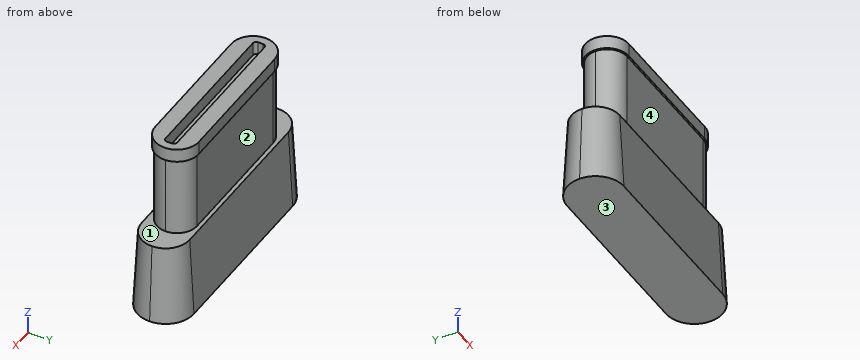
```python
from build123d import *

# Parameters (mm, degrees)
F1_DEPTH  = 2
F3_DEPTH  = 12
F5_DEPTH  = 12
F5_TAPER  = -3
F6_W      = 24
F6_H      = 1.75
F7_DEPTH  = 2
F8_R      = 0.5
F10_DEPTH = 2


with BuildPart() as f1:
    # F0 (on Top) → F1 (new body)
    with BuildSketch(Plane.XY):
        with BuildLine():
            ThreePointArc((0, 2.5), (0.732233047, 0.732233047), (2.5, 0))
            Line((2.5, 0), (22.5, 0))
            ThreePointArc((22.5, 0), (24.267766953, 0.732233047), (25, 2.5))
            ThreePointArc((25, 2.5), (24.267766953, 4.267766953), (22.5, 5))
            Line((22.5, 5), (2.5, 5))
            ThreePointArc((2.5, 5), (0.732233047, 4.267766953), (0, 2.5))
        make_face()
    extrude(amount=-F1_DEPTH)

    # F2 (on face) → F3 (join)
    with BuildSketch(Plane(origin=(0, 0, -2), x_dir=(1, 0, 0), z_dir=(0, 0, -1))):
        with BuildLine():
            ThreePointArc((2.5, 0.5), (0.3786796564, -0.3786796564), (-0.5, -2.5))
            ThreePointArc((-0.5, -2.5), (0.3786796564, -4.6213203436), (2.5, -5.5))
            Line((2.5, -5.5), (22.5, -5.5))
            ThreePointArc((22.5, -5.5), (24.6213203436, -4.6213203436), (25.5, -2.5))
            ThreePointArc((25.5, -2.5), (24.6213203436, -0.3786796564), (22.5, 0.5))
            Line((22.5, 0.5), (2.5, 0.5))
        make_face()
        with BuildLine():
            Line((2.5, 0), (22.5, 0))
            ThreePointArc((22.5, 0), (25, -2.5), (22.5, -5))
            Line((22.5, -5), (2.5, -5))
            ThreePointArc((2.5, -5), (0, -2.5), (2.5, 0))
        make_face(mode=Mode.SUBTRACT)
        with BuildLine():
            ThreePointArc((22.5, -5), (25, -2.5), (22.5, 0))
            Line((22.5, 0), (2.5, 0))
            ThreePointArc((2.5, 0), (0, -2.5), (2.5, -5))
            Line((2.5, -5), (22.5, -5))
        make_face()
    extrude(amount=F3_DEPTH)

    # F4 (on face) → F5 (join)
    with BuildSketch(Plane(origin=(0, 0, -14), x_dir=(1, 0, 0), z_dir=(0, 0, -1))):
        with BuildLine():
            Line((25.5, 1.099999994), (-0.5, 1.099999994))
            ThreePointArc((-0.5, 1.099999994), (-3.0455844081, 0.0455844081), (-4.099999994, -2.5))
            ThreePointArc((-4.099999994, -2.5), (-3.0455844081, -5.0455844081), (-0.5, -6.099999994))
            Line((-0.5, -6.099999994), (25.5, -6.099999994))
            ThreePointArc((25.5, -6.099999994), (28.0455844081, -5.0455844081), (29.099999994, -2.5))
            ThreePointArc((29.099999994, -2.5), (28.0455844081, 0.0455844081), (25.5, 1.099999994))
        make_face()
        with BuildLine():
            ThreePointArc((-3.5, -2.5), (-2.6213203436, -0.3786796564), (-0.5, 0.5))
            Line((-0.5, 0.5), (2.5, 0.5))
            Line((2.5, 0.5), (22.5, 0.5))
            Line((22.5, 0.5), (25.5, 0.5))
            ThreePointArc((25.5, 0.5), (27.6213203436, -0.3786796564), (28.5, -2.5))
            ThreePointArc((28.5, -2.5), (27.6213203436, -4.6213203436), (25.5, -5.5))
            Line((25.5, -5.5), (22.5, -5.5))
            Line((22.5, -5.5), (2.5, -5.5))
            Line((2.5, -5.5), (-0.5, -5.5))
            ThreePointArc((-0.5, -5.5), (-2.6213203436, -4.6213203436), (-3.5, -2.5))
        make_face(mode=Mode.SUBTRACT)
        with BuildLine():
            Line((22.5, 0.5), (2.5, 0.5))
            ThreePointArc((2.5, 0.5), (-0.5, -2.5), (2.5, -5.5))
            Line((2.5, -5.5), (22.5, -5.5))
            ThreePointArc((22.5, -5.5), (25.5, -2.5), (22.5, 0.5))
        make_face()
        with BuildLine():
            Line((2.5, 0.5), (-0.5, 0.5))
            ThreePointArc((-0.5, 0.5), (-2.6213203436, -0.3786796564), (-3.5, -2.5))
            ThreePointArc((-3.5, -2.5), (-2.6213203436, -4.6213203436), (-0.5, -5.5))
            Line((-0.5, -5.5), (2.5, -5.5))
            ThreePointArc((2.5, -5.5), (-0.5, -2.5), (2.5, 0.5))
        make_face()
        with BuildLine():
            Line((25.5, 0.5), (22.5, 0.5))
            ThreePointArc((22.5, 0.5), (25.5, -2.5), (22.5, -5.5))
            Line((22.5, -5.5), (25.5, -5.5))
            ThreePointArc((25.5, -5.5), (27.6213203436, -4.6213203436), (28.5, -2.5))
            ThreePointArc((28.5, -2.5), (27.6213203436, -0.3786796564), (25.5, 0.5))
        make_face()
    extrude(amount=F5_DEPTH, taper=F5_TAPER)

    # F6 (on face) → F7 (cut)
    with BuildSketch(Plane.XY):
        with Locations((12.5, 2.5)):
            Rectangle(F6_W, F6_H)
    extrude(amount=-F7_DEPTH, mode=Mode.SUBTRACT)

    # F8
    f8_edges = [f1.edges().sort_by_distance(p)[0] for p in [
        (0.5, 3.375, -1),
        (0.5, 1.625, -1),
        (24.5, 1.625, -1),
        (24.5, 3.375, -1),
    ]]
    fillet(f8_edges, radius=F8_R)

    # F9 (on face) → F10 (join)
    with BuildSketch(Plane.XY):
        with BuildLine():
            Line((22.5, 5.75), (2.5, 5.75))
            ThreePointArc((2.5, 5.75), (-0.75, 2.5), (2.5, -0.75))
            Line((2.5, -0.75), (22.5, -0.75))
            ThreePointArc((22.5, -0.75), (25.75, 2.5), (22.5, 5.75))
        make_face()
        with BuildLine():
            ThreePointArc((2.5, 0), (0, 2.5), (2.5, 5))
            Line((2.5, 5), (22.5, 5))
            ThreePointArc((22.5, 5), (25, 2.5), (22.5, 0))
            Line((22.5, 0), (2.5, 0))
        make_face(mode=Mode.SUBTRACT)
    extrude(amount=-F10_DEPTH)


solid = f1.part
```
Could you check a few things on this model? Use its own coordinates, in mm. Face numbers are marked on the shaded views. A direction names the side the tool comes from. Coordinates: 2 decimals unless noted, no trailing zeros. Write each loop counter-clockwise with the first axis right and the second up, starting at its lowest first coordinate (ties: lowest second). Pieces come first, ordered by that corner, then holes. Notation, with made-up numbers: (-11.5, 15) -> (2.5, 15) arc R6 cw to (2.5, 24) -> close; hole circle Ø11 at (-33.75, 51.5). An arc over 180 degrees is marked (long way). Return JSON: item names as keys, results as strings.
(1) Imagine slicing it at A-A, the plane z = -11.25. Please give me the cut outline in (x, y).
Numbers:
{"outline": "(2.5, -0.5) -> (22.5, -0.5) arc R3 ccw to (22.5, 5.5) -> (2.5, 5.5) arc R3 ccw to start"}
(2) Which directions (+Z, -Z, +X, -X, +Y, -Y) give clear straight access to the entire face, cutting with the end or side of a thin tool? Please do the marked faces 1 and 2.
Numbers:
{"face 1": "none", "face 2": "+X, -X, +Y"}
(3) I'm going to push flat-ended pins straight in: pin 1 (2 mm diameter, centred on x = 9, z = -1, fed in from +Y); pin 2 (0.6 mm diameter, centred on y = 2.5, z = -1, fed in from -X); pin 3 (5 mm diameter, centred on x = 23.5, z = -5.5, fed in from +Y). Where does each tip first touch, or does it pass through?
Numbers:
{"pin 1": "stops at y = 5.75", "pin 2": "stops at x = -0.75", "pin 3": "stops at y = 5.5"}
(4) We'd pull the mould along Z, two halves only. Please class the marked faces 3 and 4: +Z half, -Z half, draft (parallel to the pull), parting line (faces both ways), or undercut.
Numbers:
{"face 3": "-Z half", "face 4": "undercut"}
(5) I need wall thicknesses on L1, parallel to Y at x = 6, z = -1.5 (3 decimals); L2, parallel to Z at x = 17, y = 2.5; L3, parallel to Y at x = -3, z = -23.5. Which ranges of each line are inside material? Lowest first, please.
Numbers:
{"L1": "y = -0.75 to 1.625, 3.375 to 5.75", "L2": "z = -26 to -2", "L3": "y = -0.75 to 5.75"}
